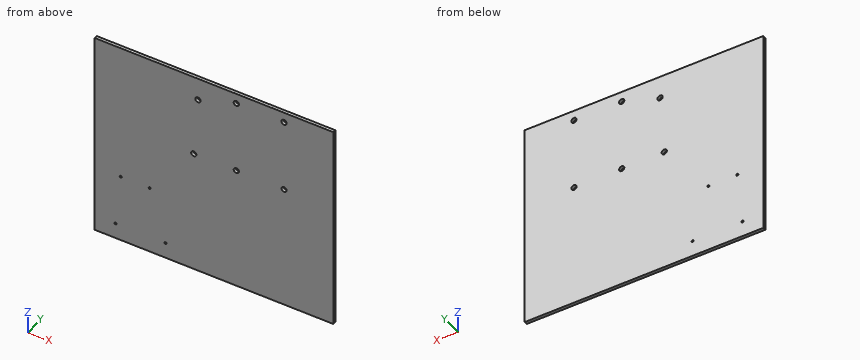
from build123d import *

# Parameters (mm, degrees)
SKETCH1_W           = 230
SKETCH1_H           = 200
SKETCH1_R           = 2.525
SKETCH1_R_2         = 1
BOSS_EXTRUDE2_DEPTH = 3


with BuildPart() as part:
    # Sketch1 → Boss-Extrude2 (new body)
    with BuildSketch(Plane(origin=(0, 0, 0), x_dir=(1, 0, 0), z_dir=(0, 1, 0))):
        with Locations((-115, 100)):
            Rectangle(SKETCH1_W, SKETCH1_H)
        with Locations(Location((-130.5, 22, 0), (0, 0, 270))):
            Circle(SKETCH1_R, mode=Mode.SUBTRACT)
        with Locations(Location((-93.5, 80, 0), (0, 0, 270))):
            Circle(SKETCH1_R, mode=Mode.SUBTRACT)
        with Locations(Location((-134.5, 80, 0), (0, 0, 270))):
            Circle(SKETCH1_R, mode=Mode.SUBTRACT)
        with Locations(Location((-47.5, 80, 0), (0, 0, 270))):
            Circle(SKETCH1_R, mode=Mode.SUBTRACT)
        with Locations(Location((-47.5, 10, 0), (0, 0, 270))):
            Circle(SKETCH1_R, mode=Mode.SUBTRACT)
        with Locations(Location((-93.5, 10, 0), (0, 0, 270))):
            Circle(SKETCH1_R, mode=Mode.SUBTRACT)
        with Locations(Location((-210, 184.76, 0), (0, 0, 270))):
            Circle(SKETCH1_R_2, mode=Mode.SUBTRACT)
        with Locations(Location((-161.74, 184.76, 0), (0, 0, 270))):
            Circle(SKETCH1_R_2, mode=Mode.SUBTRACT)
        with Locations(Location((-176.98, 133.96, 0), (0, 0, 270))):
            Circle(SKETCH1_R_2, mode=Mode.SUBTRACT)
        with Locations(Location((-204.92, 133.96, 0), (0, 0, 270))):
            Circle(SKETCH1_R_2, mode=Mode.SUBTRACT)
    extrude(amount=BOSS_EXTRUDE2_DEPTH)


solid = part.part
CAD build for the part. Positions are in the model's coordinates, mm. Round coordinates to 2 decimals unless told otherwise and drop trailing zeros. Write each loop counter-clockwise with the first axis right and the second up, starting at its lowest first coordinate (ties: lowest second). Pieces come first, ordered by that corner, then holes.
(1) Slice it at B-B, the plane x = -93.5. Write the cut outline in (y, z) (3 decimals).
(2) Slice it at A-A, the plane z = -10. Write the cut outline in (x, y) (3 decimals), and give its area (3 significant figures).
(3) Slice it at C-C, the plane z = -80. Write the cut outline in (x, y) (3 decimals), and give its area (3 significant figures).
(4) Probe line 1 along X through (y, z) = (1.3, -133.96); line 2 along X through (y, z) = (1.4, -184.76); line 3 along X through (y, z) = (1.4, -80) (3 decimals). List the from-to ranges inside material, lowest first.
From the geometry:
1. outline: (0, -200) - (3, -200) - (3, -82.525) - (0, -82.525) - close; (0, -77.475) - (3, -77.475) - (3, -12.525) - (0, -12.525) - close; (0, -7.475) - (3, -7.475) - (3, 0) - (0, 0) - close
2. outline: (-230, 0) - (-96.025, 0) - (-96.025, 3) - (-230, 3) - close; (-90.975, 0) - (-50.025, 0) - (-50.025, 3) - (-90.975, 3) - close; (-44.975, 0) - (0, 0) - (0, 3) - (-44.975, 3) - close
2. area: 660 mm2
3. outline: (-230, 0) - (-137.025, 0) - (-137.025, 3) - (-230, 3) - close; (-131.975, 0) - (-96.025, 0) - (-96.025, 3) - (-131.975, 3) - close; (-90.975, 0) - (-50.025, 0) - (-50.025, 3) - (-90.975, 3) - close; (-44.975, 0) - (0, 0) - (0, 3) - (-44.975, 3) - close
3. area: 645 mm2
4. line 1: x = -230 to -205.92, -203.92 to -177.98, -175.98 to 0
4. line 2: x = -230 to -211, -209 to -162.74, -160.74 to 0
4. line 3: x = -230 to -137.025, -131.975 to -96.025, -90.975 to -50.025, -44.975 to 0
